The listing builds one solid part. Answer for the finished solid, in the listing's coordinates (mm). Face numbers are marked on the shaded views. A direction names the side the tool comes from. Coordinates: 2 decimals unless noted, no trailing zeros. Order: outer loops, then holes, each group sorted by start corner. A loop starts at its lowest first (then second) coordinate and runs counter-clockwise, first axis right, second up.
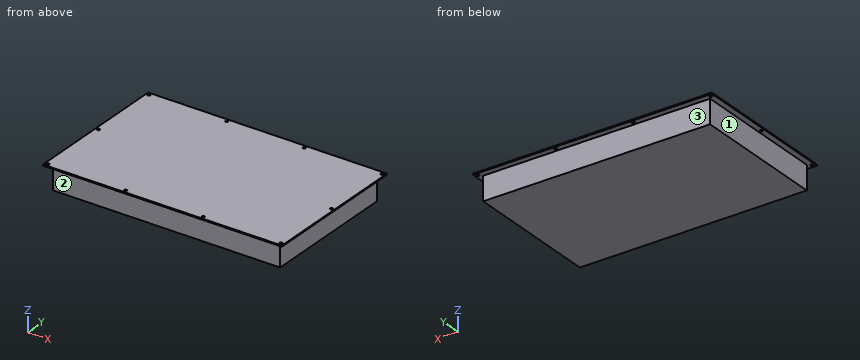
from build123d import *

# Parameters (mm, degrees)
IZIM1_W                     = 400
IZIM1_H                     = 250
Y_KSEKLIK_EKSTR_ZYON1_DEPTH = 2
KES_EKSTR_ZYON1_REACH       = 237.858
IZIM3_R                     = 2.25
IZIM4_W                     = 380
IZIM4_H                     = 230
Y_KSEKLIK_EKSTR_ZYON2_DEPTH = 40


with BuildPart() as part:
    # Çizim1 → Yükseklik-Ekstrüzyon1 (new body)
    with BuildSketch(Plane.XY):
        Rectangle(IZIM1_W, IZIM1_H)
    extrude(amount=Y_KSEKLIK_EKSTR_ZYON1_DEPTH)

    # Çizim3 → Kes-Ekstrüzyon1 (cut, up to next)
    with BuildSketch(Plane.XY.offset(2), mode=Mode.PRIVATE) as kes_ekstr_zyon1_sk1:
        with Locations((-195, 120)):
            Circle(IZIM3_R)
    kes_ekstr_zyon1_tool1 = extrude(kes_ekstr_zyon1_sk1.sketch, amount=-KES_EKSTR_ZYON1_REACH, mode=Mode.PRIVATE) & part.part
    # Çizim3 → Kes-Ekstrüzyon1 (cut, up to next)
    with BuildSketch(Plane.XY.offset(2), mode=Mode.PRIVATE) as kes_ekstr_zyon1_sk2:
        with Locations((-65, 120)):
            Circle(IZIM3_R)
    kes_ekstr_zyon1_tool2 = extrude(kes_ekstr_zyon1_sk2.sketch, amount=-KES_EKSTR_ZYON1_REACH, mode=Mode.PRIVATE) & part.part
    # Çizim3 → Kes-Ekstrüzyon1 (cut, up to next)
    with BuildSketch(Plane.XY.offset(2), mode=Mode.PRIVATE) as kes_ekstr_zyon1_sk3:
        with Locations((65, 120)):
            Circle(IZIM3_R)
    kes_ekstr_zyon1_tool3 = extrude(kes_ekstr_zyon1_sk3.sketch, amount=-KES_EKSTR_ZYON1_REACH, mode=Mode.PRIVATE) & part.part
    # Çizim3 → Kes-Ekstrüzyon1 (cut, up to next)
    with BuildSketch(Plane.XY.offset(2), mode=Mode.PRIVATE) as kes_ekstr_zyon1_sk4:
        with Locations((195, 120)):
            Circle(IZIM3_R)
    kes_ekstr_zyon1_tool4 = extrude(kes_ekstr_zyon1_sk4.sketch, amount=-KES_EKSTR_ZYON1_REACH, mode=Mode.PRIVATE) & part.part
    # Çizim3 → Kes-Ekstrüzyon1 (cut, up to next)
    with BuildSketch(Plane.XY.offset(2), mode=Mode.PRIVATE) as kes_ekstr_zyon1_sk5:
        with Locations(Location((-65, -120, 0), (0, 0, 180))):
            Circle(IZIM3_R)
    kes_ekstr_zyon1_tool5 = extrude(kes_ekstr_zyon1_sk5.sketch, amount=-KES_EKSTR_ZYON1_REACH, mode=Mode.PRIVATE) & part.part
    # Çizim3 → Kes-Ekstrüzyon1 (cut, up to next)
    with BuildSketch(Plane.XY.offset(2), mode=Mode.PRIVATE) as kes_ekstr_zyon1_sk6:
        with Locations(Location((65, -120, 0), (0, 0, 180))):
            Circle(IZIM3_R)
    kes_ekstr_zyon1_tool6 = extrude(kes_ekstr_zyon1_sk6.sketch, amount=-KES_EKSTR_ZYON1_REACH, mode=Mode.PRIVATE) & part.part
    # Çizim3 → Kes-Ekstrüzyon1 (cut, up to next)
    with BuildSketch(Plane.XY.offset(2), mode=Mode.PRIVATE) as kes_ekstr_zyon1_sk7:
        with Locations(Location((195, -120, 0), (0, 0, 180))):
            Circle(IZIM3_R)
    kes_ekstr_zyon1_tool7 = extrude(kes_ekstr_zyon1_sk7.sketch, amount=-KES_EKSTR_ZYON1_REACH, mode=Mode.PRIVATE) & part.part
    # Çizim3 → Kes-Ekstrüzyon1 (cut, up to next)
    with BuildSketch(Plane.XY.offset(2), mode=Mode.PRIVATE) as kes_ekstr_zyon1_sk8:
        with Locations(Location((-195, -120, 0), (0, 0, 180))):
            Circle(IZIM3_R)
    kes_ekstr_zyon1_tool8 = extrude(kes_ekstr_zyon1_sk8.sketch, amount=-KES_EKSTR_ZYON1_REACH, mode=Mode.PRIVATE) & part.part
    # Çizim3 → Kes-Ekstrüzyon1 (cut, up to next)
    with BuildSketch(Plane.XY.offset(2), mode=Mode.PRIVATE) as kes_ekstr_zyon1_sk9:
        with Locations(Location((-195, 0, 0), (0, 0, 180))):
            Circle(IZIM3_R)
    kes_ekstr_zyon1_tool9 = extrude(kes_ekstr_zyon1_sk9.sketch, amount=-KES_EKSTR_ZYON1_REACH, mode=Mode.PRIVATE) & part.part
    # Çizim3 → Kes-Ekstrüzyon1 (cut, up to next)
    with BuildSketch(Plane.XY.offset(2), mode=Mode.PRIVATE) as kes_ekstr_zyon1_sk10:
        with Locations(Location((195, 0, 0), (0, 0, 180))):
            Circle(IZIM3_R)
    kes_ekstr_zyon1_tool10 = extrude(kes_ekstr_zyon1_sk10.sketch, amount=-KES_EKSTR_ZYON1_REACH, mode=Mode.PRIVATE) & part.part
    add(kes_ekstr_zyon1_tool1.solids().sort_by_distance((-195, 120, 2))[0], mode=Mode.SUBTRACT)
    add(kes_ekstr_zyon1_tool2.solids().sort_by_distance((-65, 120, 2))[0], mode=Mode.SUBTRACT)
    add(kes_ekstr_zyon1_tool3.solids().sort_by_distance((65, 120, 2))[0], mode=Mode.SUBTRACT)
    add(kes_ekstr_zyon1_tool4.solids().sort_by_distance((195, 120, 2))[0], mode=Mode.SUBTRACT)
    add(kes_ekstr_zyon1_tool5.solids().sort_by_distance((-65, -120, 2))[0], mode=Mode.SUBTRACT)
    add(kes_ekstr_zyon1_tool6.solids().sort_by_distance((65, -120, 2))[0], mode=Mode.SUBTRACT)
    add(kes_ekstr_zyon1_tool7.solids().sort_by_distance((195, -120, 2))[0], mode=Mode.SUBTRACT)
    add(kes_ekstr_zyon1_tool8.solids().sort_by_distance((-195, -120, 2))[0], mode=Mode.SUBTRACT)
    add(kes_ekstr_zyon1_tool9.solids().sort_by_distance((-195, 0, 2))[0], mode=Mode.SUBTRACT)
    add(kes_ekstr_zyon1_tool10.solids().sort_by_distance((195, 0, 2))[0], mode=Mode.SUBTRACT)

    # Çizim4 → Yükseklik-Ekstrüzyon2 (add)
    with BuildSketch(Plane(origin=(0, 0, 0), x_dir=(-1, 0, 0), z_dir=(0, 0, -1))):
        Rectangle(IZIM4_W, IZIM4_H)
    extrude(amount=Y_KSEKLIK_EKSTR_ZYON2_DEPTH)


solid = part.part
(1) Given pin 1 Ø8 at (y, z) = (73.5, -30.5) entering from +X; pin 2 Ø12 at (y, z) = (33.5, -8) entering from -X; pin 3 Ø5 at (x, y) = (-195, 120) entering from -Z, each flat-ended and moving along its own axis, determine where each tip first touches the part or whether it passes through.
(2) Find the intervals of material crossed by probe 1 along Y at (x, z) = (195, 0.65); probe 2 along Y at (x, z) = (-65, 0.45); probe 3 along X at (y, z) = (-120, 0.75), in increasing order.
(3) A tool of negligible diameter and unlimited length cuts with its end or side. For the marked faces 1, 2 and 3, from which of +Z, -Z, +X, -X, +Y, -Y can it reach the whole face along a straight path? Write none if from no direction.
(4) Find section A-A on y = 81.5. Determine the outline of the cut face in (x, z).
(5) Find section C-C on z = -32. Determine the outline of the cut face in (x, y).
(6) Find section B-B on x = 150. Determine the outline of the cut face in (y, z), then the cut area to 3 significant figures.
Resolved:
1. pin 1: stops at x = 190
1. pin 2: stops at x = -190
1. pin 3: stops at z = 0
2. probe 1: y = -125 to -122.25, -117.75 to -2.25, 2.25 to 117.75, 122.25 to 125
2. probe 2: y = -125 to -122.25, -117.75 to 117.75, 122.25 to 125
2. probe 3: x = -200 to -197.25, -192.75 to -67.25, -62.75 to 62.75, 67.25 to 192.75, 197.25 to 200
3. face 1: -Z, -X, +Y, -Y
3. face 2: -Z, +X, -X, -Y
3. face 3: -Z, +X, -X, +Y
4. outline: (-200, 0) - (-190, 0) - (-190, -40) - (190, -40) - (190, 0) - (200, 0) - (200, 2) - (-200, 2) - close
5. outline: (-190, -115) - (190, -115) - (190, 115) - (-190, 115) - close
6. outline: (-125, 0) - (-115, 0) - (-115, -40) - (115, -40) - (115, 0) - (125, 0) - (125, 2) - (-125, 2) - close
6. area: 9,700 mm2
